from build123d import *

# Parameters (mm, degrees)
F0_W     = 152.4
F0_H     = 50.8
F1_DEPTH = 76.2
F2_W     = 50.8
F2_H     = 25.4
F3_DEPTH = 50.8
F4_W     = 50.8
F4_H     = 25.4
F5_DEPTH = 50.8


with BuildPart() as f1:
    # F0 (on Front) → F1 (new body)
    with BuildSketch(Plane.XZ):
        with Locations((76.2, 25.4)):
            Rectangle(F0_W, F0_H)
    extrude(amount=F1_DEPTH)

    # F2 (on face) → F3 (cut)
    with BuildSketch(Plane.XZ.offset(76.2)):
        with Locations((127, 12.7)):
            Rectangle(F2_W, F2_H)
        with Locations((127, 38.1)):
            Rectangle(F2_W, F2_H)
    extrude(amount=-F3_DEPTH, mode=Mode.SUBTRACT)

    # F4 (on face) → F5 (cut)
    with BuildSketch(Plane.YZ.offset(101.6)):
        with Locations((-50.8, 12.7)):
            Rectangle(F4_W, F4_H)
    extrude(amount=-F5_DEPTH, mode=Mode.SUBTRACT)


solid = f1.part
Verification items for the finished model (mm, model axes). A direction names the side the tool comes from. Coordinates: 2 decimals unless noted, no trailing zeros. Order: outer loops, then holes, each group sorted by start corner. A loop starts at its lowest first (then second) coordinate and runs counter-clockwise, first axis right, second up. Notation, with made-up numbers: M 46,37 L 66,37 A31 ccw 66,71 Z; hole C 82.25,-32 d3. An arc over 180 degrees is marked long. One line per item, written item: value. Start each with the question number.
Item 1: Access from +Z, -Z, +X, -X, +Y, -Y to the whole of each face (thin tool, end or side, straight path). Record for faces 1 (the flat face through (101.6, -51, 38)), 2 (the flat face through (77, -51, 25.4)), 3 (the flat face through (58, -21, 0)).
Item 2: Sectioned sample at B-B (x = 75.5). Enter the section's corners in (y, z).
Item 3: Sectioned sample at C-C (x = 141.5). Enter the section's corners in (y, z).
Item 4: Sectioned sample at A-A (z = 8). Enter the section's corners in (x, y), then the cut area to 3 significant figures.
Item 5: Gauge pin test, flat ends, axial feed: pin 1 (2 mm diameter, centred on y = -48, z = 31, fed in from +X); pin 2 (15 mm diameter, centred on x = 73.5, y = -55.5, fed in from -Z); pin 3 (2 mm diameter, centred on x = 62, z = 6, fed in from -Y). Record the tip position at first contact, or that the pin passes through.
Item 6: Scan lines: probe 1 along Y at (x, z) = (133, 14); probe 2 along X at (y, z) = (-56, 31); probe 3 along X at (y, z) = (-70, 13.5). Record each from-to range of solid material in increasing order.
Conclusion:
1. face 1: +Z, -Z, +X, -Y
1. face 2: -Z, +X, -Y
1. face 3: -Z, +X, -X, +Y, -Y
2. outline: M -76.2,25.4 L -25.4,25.4 L -25.4,0 L 0,0 L 0,50.8 L -76.2,50.8 Z
3. outline: M -25.4,0 L 0,0 L 0,50.8 L -25.4,50.8 Z
4. outline: M 0,-76.2 L 50.8,-76.2 L 50.8,-25.4 L 152.4,-25.4 L 152.4,0 L 0,0 Z
4. area: 6,450 mm^2
5. pin 1: stops at x = 101.6
5. pin 2: stops at z = 25.4
5. pin 3: stops at y = -25.4
6. probe 1: y = -25.4 to 0
6. probe 2: x = 0 to 101.6
6. probe 3: x = 0 to 50.8
